```python
from build123d import *

# Parameters (mm, degrees)
F1_DEPTH = 25.4
F2_R     = 5.08


with BuildPart() as f1:
    # F0 (on Front) → F1 (new body)
    with BuildSketch(Plane.XZ):
        Polygon((-32.336153, 17.584616), (-10.648462, 26.376924), (-10.648462, -38.295384), (-5.959231, -38.295384), (-5.959231, 50.692204), align=None)
        Polygon((-5.959231, 50.692204), (-5.959231, -38.295384), (0, -38.295384), (0, 47.434815), (-4.005384, 53.144619), align=None)
        Polygon((0, 47.434815), (0, -38.295384), (3.419231, -38.295384), (3.419231, 25.79077), (23.543846, 13.872309), align=None)
    extrude(amount=F1_DEPTH)

    # F2
    f2_edges = [f1.edges().sort_by_distance(p)[0] for p in [
        (3.419231, -25.4, -6.252307),
        (-10.648462, -25.4, -5.95923),
        (3.419231, 0, -6.252307),
        (-10.648462, 0, -5.95923),
    ]]
    fillet(f2_edges, radius=F2_R)


solid = f1.part
```
Work out the finished part from the listing and answer in its coordinate system (mm). A direction names the side the tool comes from. Coordinates: 2 decimals unless noted, no trailing zeros. Loops run counter-clockwise (first coordinate to the right, second up) from the corner with the lowest first, then second, coordinate; pieces in that order, holes last. Notation, with made-up numbers: (87, -11.75) - (145, -11.75) arc R28 ccw to (145, 16.25) - close; hole circle Ø3 at (-37.5, 49.5). An arc over 180 degrees is marked (long way). Use a Markdown table: item, result.
Item 1: The mould has two halves that part along X. Classify faces 4 (the flat face through (3.419, -13, -7)), 5 (the flat face through (-4, -13, -38.295)): +X half, -X half, draft (parallel to the pull), parting line (faces both ways), or undercut.
Evaluation:
| item | result |
|---|---|
| face 4 | undercut |
| face 5 | draft |
Item 2: For faces 1 (the cylindrical face through (1.971, -23.872, -4.278)), 2 (the cylindrical face through (1.971, -1.528, -4.278)), 3 (the flat face through (-2, 0, 21)), determine the directions among +Z, -Z, +X, -X, +Y, -Y from which every point of the face is accessible in a straight line to the end or side of a thin tool.
Evaluation:
| item | result |
|---|---|
| face 1 | -Z, -Y |
| face 2 | -Z, +Y |
| face 3 | +Z, -Z, +X, -X, +Y |
Item 3: Find section A-A, the plane y = -8.5. Determine the outline of the cut face in (x, z), and give its area (3 significant figures).
Evaluation:
| item | result |
|---|---|
| outline | (-32.34, 17.58) - (-10.65, 26.38) - (-10.65, -38.3) - (3.42, -38.3) - (3.42, 25.79) - (23.54, 13.87) - (-4.01, 53.14) - close |
| area | 1,590 mm2 |
Item 4: Consider probe 1 along X at (y, z) = (-5.25, 11.5); probe 2 along Z at (x, y) = (10, -23); probe 3 along Z at (x, y) = (16, -6.25). Determine where each line is inside the solid, lowest interval first. Write a range as from..to.
Evaluation:
| item | result |
|---|---|
| probe 1 | x = -10.65..3.42 |
| probe 2 | z = 21.89..33.18 |
| probe 3 | z = 18.34..24.63 |
Item 5: Find section D-D, the plane z = 38.5. Determine the outline of the cut face in (x, y), and give its area (3 significant figures).
Evaluation:
| item | result |
|---|---|
| outline | (-15.67, -25.4) - (6.27, -25.4) - (6.27, 0) - (-15.67, 0) - close |
| area | 557 mm2 |
Item 6: Find section B-B, the plane z = 5.5. Determine the outline of the cut face in (x, y).
Evaluation:
| item | result |
|---|---|
| outline | (-10.65, -20.32) arc R5.08 ccw to (-5.57, -25.4) - (-1.66, -25.4) arc R5.08 ccw to (3.42, -20.32) - (3.42, -5.08) arc R5.08 ccw to (-1.66, 0) - (-5.57, 0) arc R5.08 ccw to (-10.65, -5.08) - close |
Item 7: Given pin 1 Ø4.5 at (y, z) = (-11, 0.5) entering from +X; pin 2 Ø12 at (x, y) = (-23, -16.5) entering from -Z; pin 3 Ø8 at (x, z) = (-11, 15.5) entering from -Y, each flat-ended and moving along its own axis, determine where each tip first touches the part or whether it passes through.
Evaluation:
| item | result |
|---|---|
| pin 1 | stops at x = 3.42 |
| pin 2 | stops at z = 18.94 |
| pin 3 | stops at y = -25.19 |
Item 8: Find section C-C, the plane x = 6.5. Determine the outline of the cut face in (y, z).
Evaluation:
| item | result |
|---|---|
| outline | (-25.4, 23.97) - (0, 23.97) - (0, 38.17) - (-25.4, 38.17) - close |
